Job drawing, mm, ordinate dimensions from the low corner. One solid piece. A direction names the side the tool comes from. Coordinates: 2 decimals unless noted, no trailing zeros. Loops run counter-clockwise (first coordinate to the right, second up) from the corner with the lowest first, then second, coordinate; pieces in that order, holes last. Notation, with made-up numbers: M 58,13.5 L 70,13.5 A6 ccw 70,22.5 Z; hole C 34,85 d7. An arc over 180 degrees is marked long. Answer as a JSON object with one key per item and string values. Group by question number.
1. Drill centre lines: L1, parallel to Y at x = 26.5, z = 15.75; L2, parallel to X at y = 10, z = 19; L3, parallel to Z at x = 31, y = 11.5. Where is each one in solid material? Low to high.
2. Drop flat-ended pins along their axis: pin 1 Ø1 at (y, z) = (6.5, 10.5) entering from +X; pin 2 Ø3 at (x, y) = (6.5, 10.5) entering from +Z; pin 3 Ø6 at (x, y) = (31, 9) entering from +Z; pin 4 Ø1 at (y, z) = (5, 8.5) entering from -X. Give the stop position or say it passes through.
3. Saw through at A-A on z = 8. Write the cut outline in (x, y).
4. 3-axis set-ups, long thin cutter, end or side, ignore diameter. For the marked faces 1 and 2: which of +Z, -Z, +X, -X, +Y, -Y reach the whole face in a straight line?
5. Saw through at C-C on x = 37.5. Write the cut outline in (y, z), then the cut area to 3 significant figures.
6. Mould opens along Y. For the marked faces 3, 4, 5 and 6 say: released by +Y, released by -Y, zero draft, split by the parting line, or undercut.
7. Saw through at B-B on y = 2.5. Write the cut outline in (x, z), then the cut area to 4 significant figures.
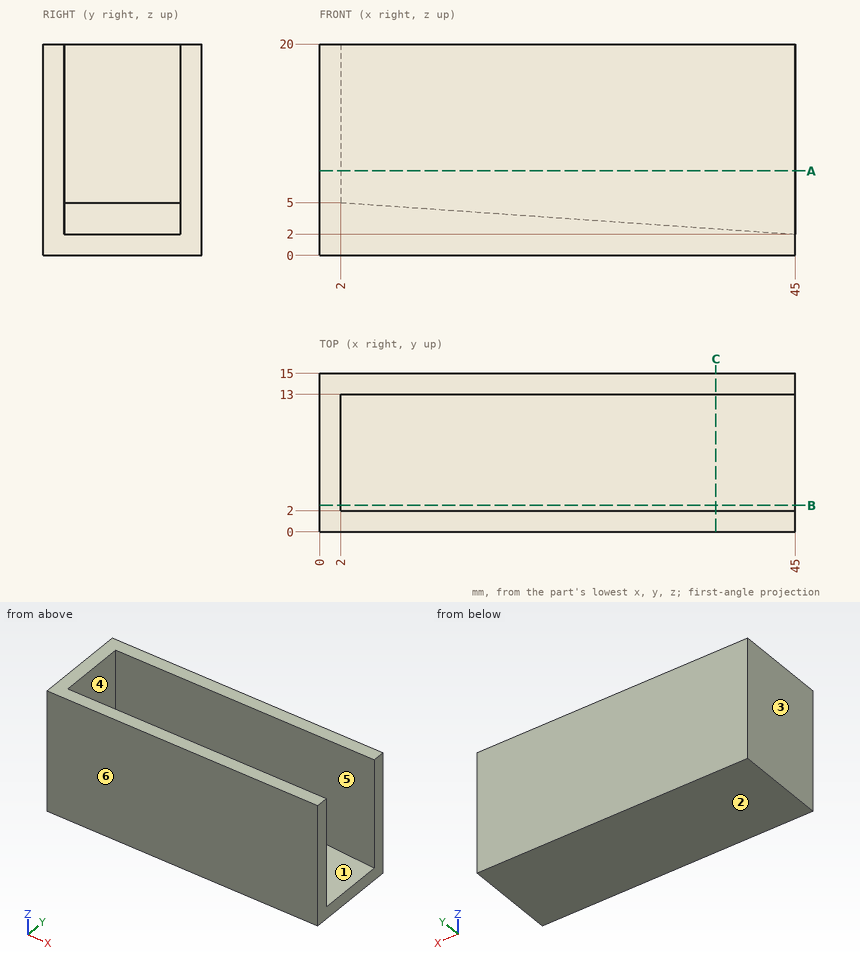
Outcome:
{
 "1": {"L1": "y = 0 to 2, 13 to 15", "L2": "x = 0 to 2", "L3": "z = 0 to 2.98"},
 "2": {"pin 1": "stops at x = 2", "pin 2": "stops at z = 4.79", "pin 3": "stops at z = 3.19", "pin 4": "stops at x = 0"},
 "3": {"outline": "M 0,0 L 45,0 L 45,2 L 2,2 L 2,13 L 45,13 L 45,15 L 0,15 Z"},
 "4": {"face 1": "+Z, +X", "face 2": "-Z, +X, -X, +Y, -Y"},
 "5": {"outline": "M 0,0 L 15,0 L 15,20 L 13,20 L 13,2.52 L 2,2.52 L 2,20 L 0,20 Z", "area": "108 mm²"},
 "6": {"face 3": "zero draft", "face 4": "undercut", "face 5": "undercut", "face 6": "released by -Y"},
 "7": {"outline": "M 0,0 L 45,0 L 45,2 L 2,5 L 2,20 L 0,20 Z", "area": "190.5 mm²"}
}
